from build123d import *

# Parameters (mm, degrees)
SKETCH3_W           = 105
SKETCH3_H           = 85
BOSS_EXTRUDE3_DEPTH = 3
SKETCH5_W           = 7
SKETCH5_H           = 7
SKETCH5_W_2         = 3
SKETCH5_H_2         = 3
BOSS_EXTRUDE4_DEPTH = 35
SKETCH9_W           = 2.998895248
SKETCH9_H           = 2.995380601
BOSS_EXTRUDE5_DEPTH = 35
SKETCH11_W          = 7
SKETCH11_H          = 7
SKETCH11_W_2        = 3
SKETCH11_H_2        = 3
BOSS_EXTRUDE6_DEPTH = 35
CUT_EXTRUDE1_DEPTH  = 6
SKETCH14_W          = 5
SKETCH14_H          = 60
CUT_EXTRUDE3_DEPTH  = 33
SKETCH17_W          = 5
SKETCH17_H          = 60
CUT_EXTRUDE4_DEPTH  = 15
SKETCH18_W          = 4
SKETCH18_H          = 4
BOSS_EXTRUDE7_DEPTH = 10


with BuildPart() as part:
    # Sketch3 → Boss-Extrude3 (new body)
    with BuildSketch(Plane(origin=(0, 0, 0), x_dir=(1, 0, 0), z_dir=(0, 1, 0))):
        with Locations((-2.316884661, -22.898810939)):
            Rectangle(SKETCH3_W, SKETCH3_H)
    extrude(amount=BOSS_EXTRUDE3_DEPTH)

    # Sketch5 → Boss-Extrude4 (add)
    with BuildSketch(Plane(origin=(0, 3, 0), x_dir=(1, 0, 0), z_dir=(0, 1, 0))):
        with Locations((11.683115339, -61.898810939)):
            Rectangle(SKETCH5_W, SKETCH5_H)
        with Locations((11.683115339, -61.898810939)):
            Rectangle(SKETCH5_W_2, SKETCH5_H_2, mode=Mode.SUBTRACT)
    extrude(amount=BOSS_EXTRUDE4_DEPTH)

    # Sketch9 → Boss-Extrude5 (add)
    with BuildSketch(Plane(origin=(0, 3, 0), x_dir=(1, 0, 0), z_dir=(0, 1, 0))):
        Polygon((15.183115339, 12.601189061), (15.183115339, 19.601189061), (8.183115339, 19.601189061), (8.183115339, 17.600348451), (8.183115339, 12.601189061), align=None)
        with Locations((11.687877227, 16.102658151)):
            Rectangle(SKETCH9_W, SKETCH9_H, mode=Mode.SUBTRACT)
    extrude(amount=BOSS_EXTRUDE5_DEPTH)

    # Sketch11 → Boss-Extrude6 (add)
    with BuildSketch(Plane(origin=(0, 3, 0), x_dir=(1, 0, 0), z_dir=(0, 1, 0))):
        with Locations((-51.316884661, -22.898810939)):
            Rectangle(SKETCH11_W, SKETCH11_H)
        with Locations((-51.316884661, -22.898810939)):
            Rectangle(SKETCH11_W_2, SKETCH11_H_2, mode=Mode.SUBTRACT)
    extrude(amount=BOSS_EXTRUDE6_DEPTH)

    # Sketch12 → Cut-Extrude1 (cut)
    with BuildSketch(Plane(origin=(0, 3, 0), x_dir=(1, 0, 0), z_dir=(0, 1, 0))):
        Polygon((29.683115339, -52.898810939), (29.683115339, -48.898810939), (29.683115339, 3.101189061), (29.683115339, 7.101189061), (24.683115339, 7.101189061), (24.683115339, -52.898810939), align=None)
    extrude(amount=-CUT_EXTRUDE1_DEPTH, mode=Mode.SUBTRACT)

    # Sketch14 → Cut-Extrude3 (cut)
    with BuildSketch(Plane(origin=(0, 3, 0), x_dir=(1, 0, 0), z_dir=(0, 1, 0))):
        with Locations((17.183115339, -22.898810939)):
            Rectangle(SKETCH14_W, SKETCH14_H)
        with Locations((-2.816884661, -22.898810939)):
            Rectangle(SKETCH14_W, SKETCH14_H)
        with Locations((-22.816884661, -22.898810939)):
            Rectangle(SKETCH14_W, SKETCH14_H)
        with Locations((-12.816884661, -22.898810939)):
            Rectangle(SKETCH14_W, SKETCH14_H)
    extrude(amount=-CUT_EXTRUDE3_DEPTH, mode=Mode.SUBTRACT)

    # Sketch17 → Cut-Extrude4 (cut)
    with BuildSketch(Plane(origin=(0, 3, 0), x_dir=(1, 0, 0), z_dir=(0, 1, 0))):
        with Locations((6.882849783, -22.898810939)):
            Rectangle(SKETCH17_W, SKETCH17_H)
    extrude(amount=-CUT_EXTRUDE4_DEPTH, mode=Mode.SUBTRACT)

    # Sketch18 → Boss-Extrude7 (add)
    with BuildSketch(Plane(origin=(0, 3, 0), x_dir=(1, 0, 0), z_dir=(0, 1, 0))):
        with Locations((31.683115339, -50.898810939)):
            Rectangle(SKETCH18_W, SKETCH18_H)
        with Locations((31.683115339, 5.101189061)):
            Rectangle(SKETCH18_W, SKETCH18_H)
        with Locations((-32.316884661, 5.101189061)):
            Rectangle(SKETCH18_W, SKETCH18_H)
        with Locations((-32.316884661, -50.898810939)):
            Rectangle(SKETCH18_W, SKETCH18_H)
    extrude(amount=BOSS_EXTRUDE7_DEPTH)


solid = part.part
Build history of the part. All positions in model axes, mm. A direction names the side the tool comes from. Coordinates: 2 decimals unless noted, no trailing zeros. Write each loop counter-clockwise with the first axis right and the second up, starting at its lowest first coordinate (ties: lowest second). Pieces come first, ordered by that corner, then holes.
(1) Cut at A-A on y = 34. List the corners of the cut face in (x, z).
(2) Cut at B-B on x = 18.5. List the corners of the cut face in (y, z).
(3) 3-axis set-ups, long thin cutter, end or side, ignore diameter. For faces 1 (the flat face through (33.683, 8, -5)), 2 (the flat face through (-32, 8, -7.101)), 3 (the flat face through (-13, 2, -7.101)), 4 (the flat face through (13.187, 20, -16)): which of +Z, -Z, +X, -X, +Y, -Y reach the whole face in a straight line?
(4) Cut at C-C on z = 4. List the corners of the cut face in (x, y).
(5) Pin check, flat tips, straight feed: pin 1 Ø6 at (x, z) = (22.5, 0.5) entering from -Y; pin 2 Ø5.5 at (x, y) = (-49.5, 18.5) entering from -Z; pin 3 Ø2 at (y, z) = (26.5, -16) entering from -X; pin 4 Ø3.5 at (y, z) = (25, 22.5) entering from +X. Stop position of each tip, or through.
(6) Drill centre lines: line 1 (Y direction, x = -6, z = -11); line 2 (X direction, y = 18, z = 24.5); line 3 (X direction, y = 20, z = 59). Where is each one in solid material? Low to high.
(7) Cut at D-D on y = 6. State how many separate pieces and enclosed holes the cut face has, and give its area (3 significant figures).
(8) Mould opens along X. For faces 5 (the flat face through (-47.817, 20, 23)), 6 (the flat face through (12, 20, 60.399)), 7 (the flat face through (32, 8, 52.899)) say: pulls with the +X half, pulls with the -X half, needs draft (parallel to the pull), parting line crosses it, or undercut.
Working result:
1. outline: (-54.82, 19.4) - (-47.82, 19.4) - (-47.82, 26.4) - (-54.82, 26.4) - close; (8.18, -19.6) - (15.18, -19.6) - (15.18, -12.6) - (8.18, -12.6) - close; (8.18, 58.4) - (15.18, 58.4) - (15.18, 65.4) - (8.18, 65.4) - close; hole (-52.82, 21.4) - (-49.82, 21.4) - (-49.82, 24.4) - (-52.82, 24.4) - close; hole (10.18, 60.4) - (13.18, 60.4) - (13.18, 63.4) - (10.18, 63.4) - close; hole (10.19, -17.6) - (13.19, -17.6) - (13.19, -14.6) - (10.19, -14.6) - close
2. outline: (0, -19.6) - (3, -19.6) - (3, -7.1) - (0, -7.1) - close; (0, 52.9) - (3, 52.9) - (3, 65.4) - (0, 65.4) - close
3. face 1: +Z, -Z, +X, +Y
3. face 2: -Z, +X, -X, +Y
3. face 3: +Y, -Y
3. face 4: +Y
4. outline: (-54.82, 0) - (-25.32, 0) - (-25.32, 3) - (-54.82, 3) - close; (-20.32, 0) - (-15.32, 0) - (-15.32, 3) - (-20.32, 3) - close; (-10.32, 0) - (-5.32, 0) - (-5.32, 3) - (-10.32, 3) - close; (-0.32, 0) - (4.38, 0) - (4.38, 3) - (-0.32, 3) - close; (9.38, 0) - (14.68, 0) - (14.68, 3) - (9.38, 3) - close; (19.68, 0) - (24.68, 0) - (24.68, 3) - (19.68, 3) - close; (29.68, 0) - (50.18, 0) - (50.18, 3) - (29.68, 3) - close
5. pin 1: stops at y = 0
5. pin 2: stops at z = 19.4
5. pin 3: stops at x = 8.18
5. pin 4: stops at x = -47.82
6. line 1: y = 0 to 3
6. line 2: x = -54.82 to -47.82
6. line 3: x = 8.18 to 15.18
7. separate pieces: 7
7. enclosed holes: 3
7. area: 184 mm2
8. face 5: pulls with the +X half
8. face 6: undercut
8. face 7: needs draft
